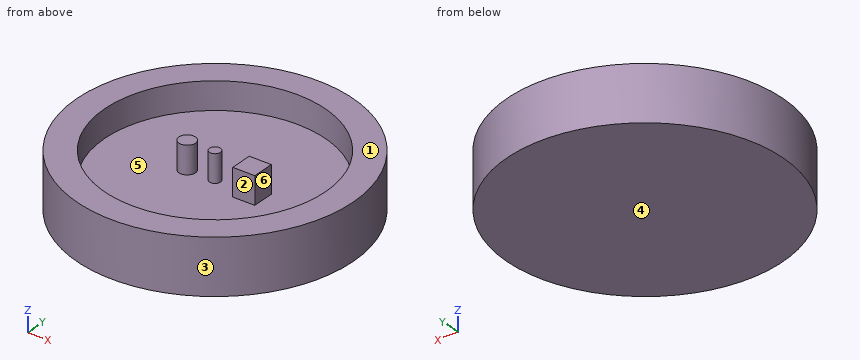
from build123d import *

# Parameters (mm, degrees)
SKETCH1_R           = 25
BOSS_EXTRUDE1_DEPTH = 10
SHELL3_T            = -5
SKETCH3_R           = 1.5
SKETCH3_R_2         = 1
SKETCH3_W           = 4
SKETCH3_H           = 4
BOSS_EXTRUDE2_DEPTH = 5


with BuildPart() as part:
    # Sketch1 → Boss-Extrude1 (new body)
    with BuildSketch(Plane.XY):
        Circle(SKETCH1_R)
    extrude(amount=BOSS_EXTRUDE1_DEPTH)

    # Shell3
    shell3_openings = [part.faces().sort_by_distance(p)[0] for p in [
        (0, 0, 10),
    ]]
    offset(amount=SHELL3_T, openings=shell3_openings, kind=Kind.INTERSECTION)

    # Sketch3 → Boss-Extrude2 (add)
    with BuildSketch(Plane.XY.offset(5)):
        with Locations((-5, -0.061087675)):
            Circle(SKETCH3_R)
        Circle(SKETCH3_R_2)
        with Locations((7, -0.381193265)):
            Rectangle(SKETCH3_W, SKETCH3_H)
    extrude(amount=BOSS_EXTRUDE2_DEPTH)


solid = part.part
Input: part model. Units: mm. Frame: model coordinates. Face numbers are marked on the shaded views. A direction names the side the tool comes from. Coordinates: 2 decimals unless noted, no trailing zeros. Loops run counter-clockwise (first coordinate to the right, second up) from the corner with the lowest first, then second, coordinate; pieces in that order, holes last. Notation, with made-up numbers: (48, 59.25) - (61, 59.25) arc R22 cw to (61, 83.25) - close; hole circle Ø10 at (14, -6). An arc over 180 degrees is marked (long way). Answer in a Markdown table with one row per item. Add a question column.
Item 1: Access query for the marked faces 1 and 2. Directions: +Z, -Z, +X, -X, +Y, -Y. A direction counts if a zero-diameter tool reaches every point of the face in a straight line with its end or side. Return the directions, or none.
Item 2: Section query D-D on x = -5. Return the cut outline in (y, z), then the cut area to 3 significant figures.
Item 3: Line query: line 1 along Y through (x, z) = (0, 8.55); line 2 along Z through (x, y) = (0, -7.5); line 3 along X through (y, z) = (-18, 8.5). Output: solid intervals per line, ascending. Write a range as [from, to].
Item 4: Section query A-A on x = 0. Return the cut outline in (y, z), then the cut area to 3 significant figures.
Item 5: Section query B-B on y = -19. Return the cut outline in (x, z) (3 decimals), then the cut area to 3 significant figures.
Item 6: Section query C-C on z = 3.25. Return the cut outline in (x, y), then the cut area to 3 significant figures.
Item 7: Mould query, pull axis Y, two halves, no side actions, for the marked faces 3, 4, 5 and 6. Classes: released by +Y, released by -Y, zero draft, split by the parting line, or undercut.
Item 8: Contact query for flat-ended pins moving along their axis: P1, Ø2, axis at x = 7, z = 7.5, coming from the +Y side; P2, Ø2, axis at x = 7.5, z = 8.5, coming from the -Y side; P3, Ø6, axis at y = -15.5, z = 2.5, coming from the +X side. Output: stop coordinate, or through.
Recorded:
| question | item | result |
|---|---|---|
| 1 | face 1 | +Z, +X, -X, +Y, -Y |
| 1 | face 2 | +Z |
| 2 | outline | (-24.49, 0) - (24.49, 0) - (24.49, 10) - (19.36, 10) - (19.36, 5) - (1.44, 5) - (1.44, 10) - (-1.56, 10) - (-1.56, 5) - (-19.36, 5) - (-19.36, 10) - (-24.49, 10) - close |
| 2 | area | 311 mm^2 |
| 3 | line 1 | [-25, -20], [-1, 1], [20, 25] |
| 3 | line 2 | [0, 5] |
| 3 | line 3 | [-17.35, -8.72], [8.72, 17.35] |
| 4 | outline | (-25, 0) - (25, 0) - (25, 10) - (20, 10) - (20, 5) - (1, 5) - (1, 10) - (-1, 10) - (-1, 5) - (-20, 5) - (-20, 10) - (-25, 10) - close |
| 4 | area | 310 mm^2 |
| 5 | outline | (-16.248, 0) - (16.248, 0) - (16.248, 10) - (6.245, 10) - (6.245, 5) - (-6.245, 5) - (-6.245, 10) - (-16.248, 10) - close |
| 5 | area | 263 mm^2 |
| 6 | outline | circle Ø50 at (0, 0) |
| 6 | area | 1,960 mm^2 |
| 7 | face 3 | split by the parting line |
| 7 | face 4 | zero draft |
| 7 | face 5 | undercut |
| 7 | face 6 | undercut |
| 8 | P1 | y = 24.27 |
| 8 | P2 | y = -24.14 |
| 8 | P3 | x = 21.65 |
